Input: part model. Units: mm. Frame: model coordinates. Face numbers are marked on the shaded views. A direction names the side the tool comes from. Coordinates: 2 decimals unless noted, no trailing zeros. Loops run counter-clockwise (first coordinate to the right, second up) from the corner with the lowest first, then second, coordinate; pieces in that order, holes last.
```python
from build123d import *

# Parameters (mm, degrees)
F0_W     = 3.048
F0_H     = 11.176
F1_DEPTH = 4.572
F2_DEPTH = 8.128
F4_DEPTH = 11.43
F5_W     = 22.86
F5_H     = 1.397
F6_DEPTH = 1.397
F7_DEPTH = 1.397


with BuildPart() as f1:
    # F0 (on Top) → F1 (new body)
    with BuildSketch(Plane.XY):
        Polygon((18.642572, -9.8425), (31.342572, -9.8425), (31.342572, -7.9375), (28.802572, -5.3975), (19.912572, -5.3975), (19.912572, 5.3975), (28.802572, 5.3975), (31.342572, 7.9375), (31.342572, 9.8425), (18.642572, 9.8425), (16.737572, 8.5725), (-23.648428, 8.5725), (-23.648428, 13.0175), (-36.348428, 13.0175), (-36.348428, 7.9375), (-42.063428, 7.9375), (-51.842428, -7.9375), (-36.348428, -7.9375), (-36.348428, -13.0175), (-23.648428, -13.0175), (-23.648428, -8.5725), (16.737572, -8.5725), align=None)
        with BuildLine():
            Line((-32.792428, 5.08), (-20.092428, 5.08))
            ThreePointArc((-20.092428, 5.08), (-15.012428, 0), (-20.092428, -5.08))
            Line((-20.092428, -5.08), (-32.792428, -5.08))
            ThreePointArc((-32.792428, -5.08), (-37.872428, 0), (-32.792428, 5.08))
        make_face(mode=Mode.SUBTRACT)
        with Locations((-1.423428, 0)):
            Rectangle(F0_W, F0_H, mode=Mode.SUBTRACT)
    extrude(amount=F1_DEPTH)

    # F0 (on Top) → F2 (join)
    with BuildSketch(Plane.XY):
        with Locations((-1.423428, 0)):
            Rectangle(F0_W, F0_H)
    extrude(amount=F2_DEPTH)

    # F3 (on face) → F4 (join)
    with BuildSketch(Plane.YZ.offset(-23.648428)):
        with BuildLine():
            ThreePointArc((-10.733225, 0), (-9.69486, 0.467551), (-9.269748, 1.524))
            ThreePointArc((-9.269748, 1.524), (-11.851449, 2.62414), (-10.856775, 0))
            Line((-10.856775, 0), (-10.733225, 0))
        make_face()
    extrude(amount=F4_DEPTH)

    # F5 (on face) → F6 (cut)
    with BuildSketch(Plane(origin=(0, 0, 0), x_dir=(1, 0, 0), z_dir=(0, 0, -1))):
        with Locations((5.307572, 7.874)):
            Rectangle(F5_W, F5_H)
    extrude(amount=-F6_DEPTH, mode=Mode.SUBTRACT)

    # F5 (on face) → F7 (cut)
    with BuildSketch(Plane(origin=(0, 0, 0), x_dir=(1, 0, 0), z_dir=(0, 0, -1))):
        with Locations((5.307572, -7.874)):
            Rectangle(F5_W, F5_H)
    extrude(amount=-F7_DEPTH, mode=Mode.SUBTRACT)


solid = f1.part
```
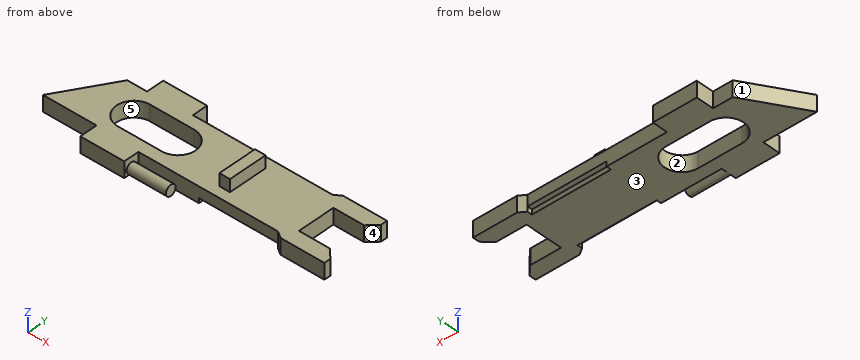
Item 1: Mould query, pull axis Y, two halves, no side actions, for the marked faces 1, 2 and 3. Classes: +Y half, -Y half, draft (parallel to the pull), parting line (faces both ways), or undercut.
Result:
face 1: +Y half
face 2: undercut
face 3: draft
Item 2: Reachability of the marked faces 4 and 5 from +Z, -Z, +X, -X, +Y, -Y: full face, straight path, thin tool, end or side. Return the list, or none.
Result:
face 4: +Z, -Z, +X
face 5: +Z, -Z
Item 3: Section query A-A (y = 3.5). Output: boundary loops of the cut face in (x, z), then the cut area to 3 significant figures.
Result:
outline: (-44.8, 0) - (-36.47, 0) - (-36.47, 4.57) - (-44.8, 4.57) - close; (-16.41, 0) - (19.91, 0) - (19.91, 4.57) - (0.1, 4.57) - (0.1, 8.13) - (-2.95, 8.13) - (-2.95, 4.57) - (-16.41, 4.57) - close
area: 215 mm2
Item 4: Contact query for flat-ended pins moving along their axis: P1, Ø3, axis at y = -2, z = 6, coming from the +X side; P2, Ø1.5, axis at y = 8, z = 0.5, coming from the -X side; P3, Ø2.5, axis at x = 25.5, z = 3, coming from the -Y side. Output: stop coordinate, or through.
Result:
P1: stops at x = 19.91
P2: stops at x = -42.49
P3: stops at y = -9.84
Item 5: Line query: L1, parallel to Y at x = 25, z = 4; L2, parallel to X at y = 1.75, z = 4.75; L3, parallel to Y at x = -41.5, z = 4. Output: solid intervals per line, ascending.
Result:
L1: y = -9.84 to -5.4, 5.4 to 9.84
L2: x = -2.95 to 0.1
L3: y = -7.94 to 7.94
Item 6: Section query B-B (x = 15.5). Output: boundary loops of the cut face in (y, z), then the cut area to 3 significant figures.
Result:
outline: (-8.57, 1.4) - (-7.18, 1.4) - (-7.18, 0) - (7.18, 0) - (7.18, 1.4) - (8.57, 1.4) - (8.57, 4.57) - (-8.57, 4.57) - close
area: 74.5 mm2
Item 7: Section query D-D (x = -17). Count the separate pieces of the cut face and the enclosed holes in it, then the cut area to 3 significant figures.
Result:
separate pieces: 3
enclosed holes: 0
area: 48.8 mm2
